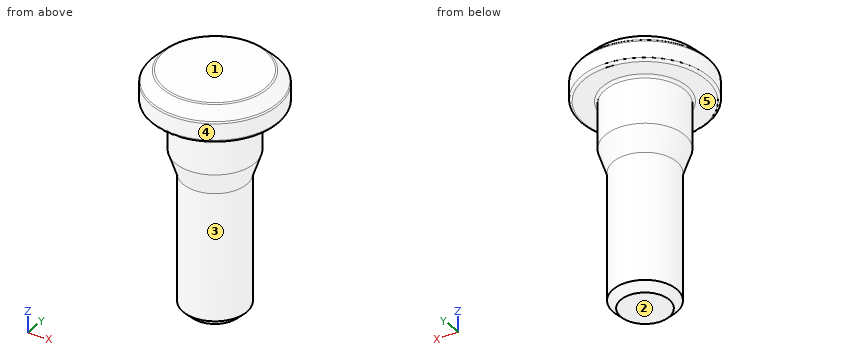
```python
from build123d import *

# Parameters (mm, degrees)
FILLET1_R = 0.508


with BuildPart() as part:
    # Sketch1 → Base-Revolve (revolve)
    with BuildSketch(Plane(origin=(0, 0, 0), x_dir=(0, 0, -1), z_dir=(1, 0, 0)), mode=Mode.PRIVATE) as base_revolve_sk:
        Polygon((-6.35, 0), (41.275, 0), (41.275, 4.826), (39.751, 6.35), (14.2875, 6.35), (9.525, 7.9375), (0, 7.9375), (0, 12.7), (-3.9878, 12.7), (-6.35, 10.3378), align=None)
    revolve(base_revolve_sk.sketch.rotate(Axis((0, 0, 0), (0, 0, 1)), 90), axis=Axis((0, 0, 0), (0, 0, 1)))

    # Fillet1
    fillet1_edges = [part.edges().sort_by_distance(p)[0] for p in [
        (7.9375, 0, 0),
        (12.7, 0, 0),
        (12.7, 0, 3.9878),
        (10.3378, 0, 6.35),
    ]]
    fillet(fillet1_edges, radius=FILLET1_R)


solid = part.part
```
Could you check a few things on this model? Use its own coordinates, in mm. Face numbers are marked on the shaded views. A direction names the side the tool comes from. Round coordinates to 2 decimals unless told otherwise and drop trailing zeros. Loops run counter-clockwise (first coordinate to the right, second up) from the corner with the lowest first, then second, coordinate; pieces in that order, holes last. Notation, with made-up numbers: (-14.5, 83) - (28.5, 83) arc R22 ccw to (28.5, 122) - close; hole circle Ø1 at (74.25, 39.25). An arc over 180 degrees is marked (long way). Use CSV: the item, a comma, the result in double quotes.
Item 1: If we mould it in two halves opening along Z, with no side actions, what happens to the marked faces 1, 2 and 3? For each: pulls with the +Z half, pulls with the -Z half, needs draft (parallel to the pull), parting line crosses it, or undercut.
Here are the results:
face 1,"pulls with the +Z half"
face 2,"pulls with the -Z half"
face 3,"needs draft"
Item 2: If we section it at A-A on z = -30: List the corners of the cut face in (x, y) for me, then the cut area to 3 significant figures.
Here are the results:
outline,"circle Ø12.7 at (0, 0)"
area,"127 mm²"
Item 3: If we section it at B-B on z = -7.5: List the corners of the cut face in (x, y) for me (1 decimal).
Here are the results:
outline,"circle Ø15.9 at (0, 0)"
Item 4: I need wall thicknesses on L1, parallel to Z at x = -2.75, y = -9.25; L2, parallel to Y at x = 3.5, z = -1; L3, parallel to Z at x = 5.75, y = 2. Which ranges of each line are inside material? Lowest first, please. Write a range as [from, to].
Here are the results:
L1,"z = [0, 6.35]"
L2,"y = [-7.12, 7.12]"
L3,"z = [-40.01, 6.35]"
Item 5: For the marked faces 4 and 5, which set-ups out of +Z, -Z, +X, -X, +Y, -Y let a thin tool reach every point of the face, with its end or its side?
Here are the results:
face 4,"+Z, -Z"
face 5,"-Z"
Item 6: Will these pins go through, and if not, where does the flat tip stop? pin 1 (8 mm diameter, centred on y = 1.5, z = -14.5, fed in from +X); pin 2 (3 mm diameter, centred on y = 7.5, z = -6.5, fed in from +X); pin 3 (6 mm diameter, centred on y = 6, z = -13.5, fed in from -X); pin 4 (1 mm diameter, centred on y = 8.5, z = -16, fed in from +X).
Here are the results:
pin 1,"stops at x = 7.55"
pin 2,"stops at x = 5.2"
pin 3,"stops at x = -6.25"
pin 4,"passes through"
